Autodesk Inventor part; units mm, degrees
ref_plane "YZ Plane" through (0, 0, 0) normal (1, 0, 0) x (0, 1, 0)
ref_plane "XZ Plane" through (0, 0, 0) normal (0, 1, 0) x (-1, 0, 0)
ref_plane "XY Plane" through (0, 0, 0) normal (0, 0, 1) x (1, 0, 0)
sketch "Sketch1" plane through (0, 0, 0) normal (1, 0, 0) x (0, 1, 0)
  point P0 (0, 0)
sketch "Sketch2" plane through (0, 0, 0) normal (1, 0, 0) x (0, 1, 0)
  line L0 (0, 0) -> (-18, 0)
  line L1 (-18, 0) -> (-18, -50)
  line L2 (0, -50) -> (0, 0)
  arc A0 (-18, -50) -> (0, -50) centre (-9, -50) ccw
  point P0 (-4.8185, -57.9696)
  dimension "d0" = 18
  dimension "d1" = 50
  dimension "d4" = 18
extrude "Extrusion1" add sketch "Sketch2" along normal blind 5
sketch "Sketch3" plane through (5, 0, 0) normal (1, 0, 0) x (0, 0, -1)
  arc A0 (50, -18) -> (50, 0) centre (50, -9) ccw
  circle A1 centre (50, -9) radius 3.1
  arc A2 (10, -5.9) -> (10, -12.1) centre (10, -9) ccw
  arc A3 (30, -12.1) -> (30, -5.9) centre (30, -9) ccw
  line L0 (10, -5.9) -> (30, -5.9)
  line L1 (10, -12.1) -> (30, -12.1)
  line L2 (0, 0) -> (0, -18)
  dimension "d5" = 6.2
  dimension "d6" = 6.2
  dimension "d7" = 6.2
  dimension "d8" = 10
  dimension "d9" = 20
extrude "Extrusion2" cut sketch "Sketch3" against normal through all
properties part number "roller bracket"
Here's how the part is built. I have some questions about the finished solid (model axes, mm). A direction names the side the tool comes from. Coordinates: 2 decimals unless noted, no trailing zeros. Loops run counter-clockwise (first coordinate to the right, second up) from the corner with the lowest first, then second, coordinate; pieces in that order, holes last. Notation, with made-up numbers: (-31, 84.5) -> (15, 84.5) arc R19 ccw to (15, 112.5) -> close; hole circle Ø11 at (58, 21.5). An arc over 180 degrees is marked (long way). Use one line per item in the form item = value. Start each with the question number.
(1) If we section it at B-B (y = -9): Please give me the cut outline in (x, z), then the cut area to 3 significant figures.
(2) Please list where these lines run through material, in increasing order: line 1 along Z through (x, y) = (0.75, -9.25); line 2 along Y through (x, z) = (1.25, -50); line 3 along Z through (x, y) = (0.8, -6.5).
(3) On a 3-axis mill with a long thin cutter (end or side, diameter ignored), from which of +Z, -Z, +X, -X, +Y, -Y can I reach the whole of each face in a straight line? I mean faces 4 (the face through (0, -5, -29)), 5 (the face through (3, -5.9, -20)). Say none if no direction works.
(4) If we section it at A-A (x = 1.6): Please give me the cut outline in (y, z).
(5) If we section it at C-C (y = -4.5): Please give me the cut outline in (x, z), then the cut area to 3 significant figures.
(6) If we section it at D-D (y = -15.5): Please give me the cut outline in (x, z), then the cut area to 3 significant figures.
(7) Will these pins go through, and if not, where does the flat tip stop? pin 1 (1 mm diameter, centred on x = 1.5, y = -7, fed in from +Z); pin 2 (1 mm diameter, centred on y = -7, z = -50.5, fed in from +X).
(8) We'd pull the mould along Z, two halves only. Please class faces 1 (the face through (2, -9, -59)), 2 (the face through (2, -18, -25)), 3 (the face through (2.535, -5.926, -49.596)): pulls with the +Z half, pulls with the -Z half, needs draft (parallel to the pull), parting line crosses it, or undercut.
Verdict:
q1.outline = (0, -59) -> (5, -59) -> (5, -53.1) -> (0, -53.1) -> close; (0, -46.9) -> (5, -46.9) -> (5, -33.1) -> (0, -33.1) -> close; (0, -6.9) -> (5, -6.9) -> (5, 0) -> (0, 0) -> close
q1.area = 133 mm²
q2.line_1 = -59 to -53.09, -46.91 to -33.09, -6.91 to 0
q2.line_2 = -18 to -12.1, -5.9 to 0
q2.line_3 = -58.65 to -51.83, -48.17 to -31.83, -8.17 to 0
q3.face_4 = +Z, -Z, -X, +Y, -Y
q3.face_5 = +X, -X
q4.outline = (-18, -50) arc R9 ccw to (0, -50) -> (0, 0) -> (-18, 0) -> close; hole circle Ø6.2 at (-9, -50); hole (-12.1, -30) arc R3.1 ccw to (-5.9, -30) -> (-5.9, -10) arc R3.1 ccw to (-12.1, -10) -> close
q5.outline = (0, -57.79) -> (5, -57.79) -> (5, 0) -> (0, 0) -> close
q5.area = 289 mm²
q6.outline = (0, -56.22) -> (5, -56.22) -> (5, 0) -> (0, 0) -> close
q6.area = 281 mm²
q7.pin_1 = 0
q7.pin_2 = through
q8.face_1 = pulls with the -Z half
q8.face_2 = needs draft
q8.face_3 = undercut
